```python
from build123d import *

# Parameters (mm, degrees)
F1_DEPTH = 4
F2_R     = 5.9436
F2_R_2   = 1.6637
F2_R_3   = 1.5875
F3_DEPTH = 25
F4_R     = 5
F5_R     = 2
F6_SIZE  = 3
F7_SIZE  = 3


# Not quite as in the source:
# - a feature names something its author has since deleted; it is built from what else it names


with BuildPart() as f1:
    # F0 (on Top) → F1 (new body)
    with BuildSketch(Plane.XY):
        Polygon((65, -25), (65, 25), (33, 25), (-33, 25), (-65, 25), (-65, -25), align=None)
    extrude(amount=F1_DEPTH)

    # F2 (on Top) → F3 (cut)
    with BuildSketch(Plane.XY):
        with Locations((-25, 0)):
            Circle(F2_R)
        Circle(F2_R_2)
        with Locations((25, 0)):
            Circle(F2_R)
        with Locations((-56.9125, 13.4125)):
            Circle(F2_R_3)
        with Locations((-56.9125, -13.4125)):
            Circle(F2_R_3)
        with Locations((56.9125, 13.4125)):
            Circle(F2_R_3)
        with Locations((56.9125, -13.4125)):
            Circle(F2_R_3)
    extrude(amount=F3_DEPTH, mode=Mode.SUBTRACT)

    # F4
    f4_edges = [f1.edges().sort_by_distance(p)[0] for p in [
        (-65, -25, 2),
        (65, -25, 2),
        (65, 25, 2),
        (-65, 25, 2),
    ]]
    fillet(f4_edges, radius=F4_R)

    # F5
    f5_edges = [f1.edges().sort_by_distance(p)[0] for p in [
        (-65, 0, 4),
    ]]
    fillet(f5_edges, radius=F5_R)

    # F6
    f6_edges = [f1.edges().sort_by_distance(p)[0] for p in [
        (-30.9436, 0, 4),
        (19.0564, 0, 4),
    ]]
    chamfer(f6_edges, length=F6_SIZE)

    # F7
    f7_edges = [f1.edges().sort_by_distance(p)[0] for p in [
        (-1.6637, 0, 4),
    ]]
    chamfer(f7_edges, length=F7_SIZE)


solid = f1.part
```
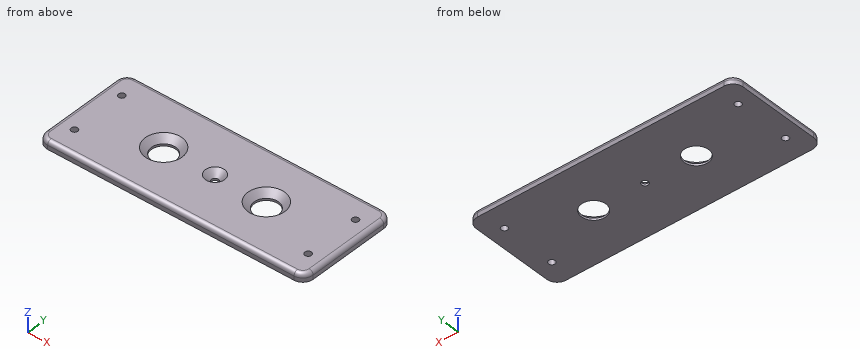
Geometry: final body of the model. Coordinates: model frame, mm. Coordinates: 2 decimals unless noted, no trailing zeros. Write each loop counter-clockwise with the first axis right and the second up, starting at its lowest first coordinate (ties: lowest second). Pieces come first, ordered by that corner, then holes. Notation, with made-up numbers: M -31.5,12 L 20.5,12 A32 ccw 20.5,44 Z; hole C -9,81 d9. An arc over 180 degrees is marked long. Use CSV: the item, a comma, the result in double quotes. Start each with the question number.
1. Ray query, probe 1 along X at (y, z) = (0, 0.8); probe 2 along Y at (x, z) = (-25, 0.5); probe 3 along X at (y, z) = (2.5, 1.25). Return the intervals inside material, ascending.
2. Cut plane C-C on z = 3.2. Return the cut outline in (x, y) (1 decimal), plus the area to 3 significant figures.
3. Cut plane D-D on x = -25. Return the cut outline in (y, z), plus the area to 3 significant figures.
4. Cut plane A-A on x = 0. Return the cut outline in (y, z).
5. Cut plane B-B on y = 0. Return the cut outline in (x, z).
6. First-contact query: P1, Ø1.5, axis at y = -2.5, z = 3, coming from the -X side; P2, Ø4, axis at x = 0, y = 0, coming from the +Z side. Flat tips, straight axial feed; report the tip coordinate or a pass-through.
Entries:
1,probe 1,"-65 to -30.94, -19.06 to -1.66, 1.66 to 19.06, 30.94 to 65"
1,probe 2,"-25 to -5.94, 5.94 to 25"
1,probe 3,"-65 to -30.67, -19.33 to 19.33, 30.67 to 65"
2,outline,"M -64.6,-20 A4.6 ccw -60,-24.6 L 60,-24.6 A4.6 ccw 64.6,-20 L 64.6,20 A4.6 ccw 60,24.6 L -60,24.6 A4.6 ccw -64.6,20 Z; hole C -56.9,-13.4 d3.2; hole C -56.9,13.4 d3.2; hole C -25,0 d16.3; hole C 0,0 d7.7; hole C 25,0 d16.3; hole C 56.9,-13.4 d3.2; hole C 56.9,13.4 d3.2"
2,area,"5,840 mm²"
3,outline,"M -25,0 L -5.94,0 L -5.94,1 L -8.94,4 L -23,4 A2 ccw -25,2 Z; M 5.94,0 L 25,0 L 25,2 A2 ccw 23,4 L 8.94,4 L 5.94,1 Z"
3,area,"142 mm²"
4,outline,"M -25,0 L -1.66,0 L -1.66,1 L -4.66,4 L -23,4 A2 ccw -25,2 Z; M 1.66,0 L 25,0 L 25,2 A2 ccw 23,4 L 4.66,4 L 1.66,1 Z"
5,outline,"M -65,0 L -30.94,0 L -30.94,1 L -33.94,4 L -63,4 A2 ccw -65,2 Z; M -19.06,0 L -1.66,0 L -1.66,1 L -4.66,4 L -16.06,4 L -19.06,1 Z; M 1.66,0 L 19.06,0 L 19.06,1 L 16.06,4 L 4.66,4 L 1.66,1 Z; M 30.94,0 L 65,0 L 65,2 A2 ccw 63,4 L 33.94,4 L 30.94,1 Z"
6,P1,"x = -64.98"
6,P2,"z = 1.34"
